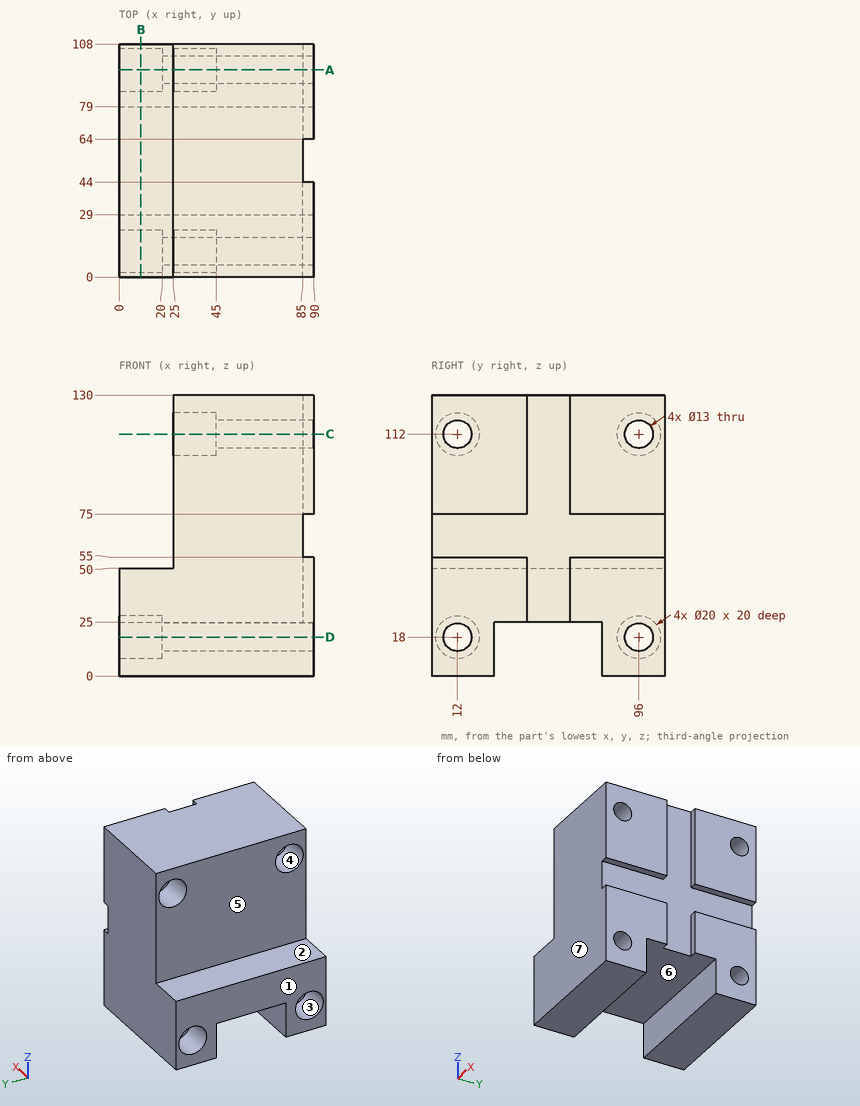
Here's the drawing with two shaded views (mm, measured from the low corner). I have some questions. A direction names the side the tool comes from. Give positions to 0.01 mm unless a question says otherwise; leave off trailing zeros. Order: outer loops, then holes, each group sorted by start corner. A loop starts at its lowest first (then second) coordinate and runs counter-clockwise, first axis right, second up. Notation, with made-up numbers: M 26,89 L 31,89 A25 cw 31,114 Z; hole C 3.5,-37 d9. An arc over 180 degrees is marked long. One line per question, with ' | ' between items.
Item 1: Suppose I cut it at A-A, the plane y = 96. Write out the boundary of the cut face in (x, z).
Answer block:
outline: M 0,0 L 90,0 L 90,11.5 L 20,11.5 L 20,8 L 0,8 Z; M 0,28 L 20,28 L 20,24.5 L 90,24.5 L 90,55 L 85,55 L 85,75 L 90,75 L 90,105.5 L 45,105.5 L 45,102 L 25,102 L 25,50 L 0,50 Z; M 25,122 L 45,122 L 45,118.5 L 90,118.5 L 90,130 L 25,130 Z
Item 2: I'm going to push flat-ended pins straight in: pin 1 Ø18 at (y, z) = (96, 18) entering from -X; pin 2 Ø7.5 at (x, y) = (12.5, 69) entering from +Z; pin 3 Ø5 at (x, y) = (77, 32.5) entering from -Z. Where does each tip first touch, or does it pass through?
Answer block:
pin 1: stops at x = 20 | pin 2: stops at z = 50 | pin 3: stops at z = 25
Item 3: Suppose I cut it at B-B, the plane x = 10. Write out the boundary of the cut face in (y, z).
Answer block:
outline: M 0,0 L 29,0 L 29,25 L 79,25 L 79,0 L 108,0 L 108,50 L 0,50 Z; hole C 12,18 d20; hole C 96,18 d20
Item 4: Please list where these lines run through material, in increasing order: L1, parallel to Y at x = 66, z = 112; L2, parallel to Z at x = 36, y = 12; L3, parallel to Z at x = 66, y = 96.
Answer block:
L1: y = 0 to 5.5, 18.5 to 89.5, 102.5 to 108 | L2: z = 0 to 11.5, 24.5 to 102, 122 to 130 | L3: z = 0 to 11.5, 24.5 to 105.5, 118.5 to 130
Item 5: Suppose I cut it at C-C, the plane z = 112. Write out the boundary of the cut face in (x, y).
Answer block:
outline: M 25,0 L 90,0 L 90,5.5 L 45,5.5 L 45,2 L 25,2 Z; M 25,22 L 45,22 L 45,18.5 L 90,18.5 L 90,44 L 85,44 L 85,64 L 90,64 L 90,89.5 L 45,89.5 L 45,86 L 25,86 Z; M 25,106 L 45,106 L 45,102.5 L 90,102.5 L 90,108 L 25,108 Z
Item 6: Suppose I cut it at D-D, the plane z = 18. Write out the boundary of the cut face in (x, y).
Answer block:
outline: M 0,0 L 90,0 L 90,5.5 L 20,5.5 L 20,2 L 0,2 Z; M 0,22 L 20,22 L 20,18.5 L 90,18.5 L 90,29 L 0,29 Z; M 0,79 L 90,79 L 90,89.5 L 20,89.5 L 20,86 L 0,86 Z; M 0,106 L 20,106 L 20,102.5 L 90,102.5 L 90,108 L 0,108 Z
Item 7: For the marked faces 4, 5, 6 and 7, which set-ups out of +Z, -Z, +X, -X, +Y, -Y let a thin tool reach every point of the face, with its end or its side?
Answer block:
face 4: -X | face 5: +Z, -X, +Y, -Y | face 6: -Z, +X, -X | face 7: +Z, -Z, +X, -X, -Y
Item 8: We'd pull the mould along Z, two halves only. Please class the marked faces 1, 2 and 3: released by +Z, released by -Z, zero draft, split by the parting line, or undercut.
Answer block:
face 1: zero draft | face 2: released by +Z | face 3: undercut
